Read the model definition and answer for the solid it produces. Units are mm, in the model's axes. A direction names the side the tool comes from. Coordinates: 2 decimals unless noted, no trailing zeros. Write each loop counter-clockwise with the first axis right and the second up, starting at its lowest first coordinate (ties: lowest second). Pieces come first, ordered by that corner, then holes.
(1) Find the intervals of material crossed by probe 1 along X at (y, z) = (34.5, -19.5); probe 2 along Z at (x, y) = (18.5, 43); probe 3 along X at (y, z) = (32, -22.5), in increasing order.
(2) Section C-C on y = 27 is taken. Write down the section's boundary in (x, z).
(3) Section A-A on y = -19 is taken. Write down the section's boundary in (x, z), then the cut area to 3 significant figures.
(4) Which of the six approach directions +Z, -Z, +X, -X, +Y, -Y give full straight-line access (tool end or side, diameter ignored) to faces 4 (the flat face through (11, -5, -36)), 5 (the flat face through (17.5, 0, 2)), 6 (the flat face through (22.56, 22.88, -23.2)), 7 (the cylindrical face through (12.99, -20.72, 1.52)), 8 (the flat face through (-1, 47, 13))?
(5) The mould has two halves that part along X. Classify faces 1 (the flat face through (50, 8, 1)), 2 (the flat face through (-17.5, 0, 2)), 3 (the flat face through (-50, 11, 2)): +X half, -X half, draft (parallel to the pull), parting line (faces both ways), or undercut.
(6) Section D-D on z = -21 is taken. Write down the section's boundary in (x, y).
(7) Section B-B on x = -15 is taken. Write down the section's boundary in (y, z), then the cut area to 3 significant figures.
(8) Given pin 1 (15 mm diameter, centred on x = 5, z = -36.5, fed in from -Y); pin 2 (10 mm diameter, centred on x = 22.5, z = 10.5, fed in from -Y); pin 3 (5 mm diameter, centred on x = -22.5, y = 15.5, fed in from -Z); pin 4 (12 mm diameter, centred on x = 18, z = -14.5, fed in from +Y), each flat-ended and moving along its own axis, determine where each tip first touches the part or whether it passes through.
Autodesk Inventor part; units mm, degrees
ref_plane "YZ Plane" through (0, 0, 0) normal (1, 0, 0) x (0, 1, 0)
ref_plane "XZ Plane" through (0, 0, 0) normal (0, 1, 0) x (-1, 0, 0)
ref_plane "XY Plane" through (0, 0, 0) normal (0, 0, 1) x (1, 0, 0)
sketch "Sketch1" plane through (0, 0, 0) normal (0, 0, 1) x (1, 0, 0)
  line L0 (-50, -50) -> (50, -50)
  line L1 (50, -50) -> (50, 50)
  line L2 (50, 50) -> (-50, 50)
  line L3 (-50, 50) -> (-50, -50)
  line L4 (-50, -50) -> (50, 50) construction
  line L5 (50, -50) -> (-50, 50) construction
  point P0 (0, 0)
  dimension "d0" = 100
  dimension "d1" = 100
extrude "Extrusion1" add sketch "Sketch1" along normal blind 3
sketch "Sketch2" plane through (-50, 50, 0) normal (0, 1, 0) x (1, 0, 0)
  line L0 (0, 0) -> (100, 0)
  line L1 (0, 0) -> (50, 50)
  line L2 (50, 50) -> (52.1213, 47.8787)
  line L3 (52.1213, 47.8787) -> (2.1213, -2.1213)
  line L4 (2.1213, -2.1213) -> (0, 0)
  line L5 (0, 0) -> (70.7107, 0) construction
  line L6 (100, 0) -> (52.1213, 47.8787)
  line L7 (52.1213, 47.8787) -> (50, 45.7574)
  line L8 (50, 45.7574) -> (97.8787, -2.1213)
  line L9 (97.8787, -2.1213) -> (100, 0)
  point P0 (50, 0)
  dimension "d4" = 45
  dimension "d5" = 3
  dimension "d6" = 3
extrude "Extrusion2" add sketch "Sketch2" against normal blind 55 contours L1 L2 L3 L0 | L0 L3 L4 | L8 L3 L6 L0 | L0 L9 L8
sketch "Sketch3" plane through (0, 0, 3) normal (0, 0, 1) x (1, 0, 0)
  line L0 (2.5, -25) -> (-2.5, -25)
  line L1 (-17.5, -10) -> (-17.5, 10)
  line L2 (-2.5, 25) -> (2.5, 25)
  line L3 (17.5, 10) -> (17.5, -10)
  line L4 (17.5, -25) -> (-17.5, 25) construction
  line L5 (-17.5, -25) -> (17.5, 25) construction
  arc A0 (-2.5, 25) -> (-17.5, 10) centre (-2.5, 10) ccw
  arc A1 (17.5, 10) -> (2.5, 25) centre (2.5, 10) ccw
  arc A2 (2.5, -25) -> (17.5, -10) centre (2.5, -10) ccw
  arc A3 (-17.5, -10) -> (-2.5, -25) centre (-2.5, -10) ccw
  point P0 (0, 0)
  dimension "d9" = 35
  dimension "d10" = 50
  dimension "d11" = 15
extrude "Extrusion3" cut sketch "Sketch3" against normal blind 3
sketch "Sketch5" plane through (-50, 50, 3) normal (0, 1, 0) x (1, 0, 0)
  line L0 (0, 3) -> (0, 0)
  line L1 (0, 0) -> (100, 0)
  line L2 (100, 0) -> (100, -20)
  line L3 (100, -20) -> (0, -20)
  line L4 (0, -20) -> (0, 0)
  point P0 (50, 3)
  dimension "d16" = 100
  dimension "d17" = 20
extrude "Extrusion5" add sketch "Sketch5" against normal blind 3
properties part number "fixation_v02"
Response:
1. probe 1: x = -30.5 to -26.26, 26.26 to 30.5
1. probe 2: z = -31.5 to -27.26, 0 to 3
1. probe 3: x = -27.5 to -23.26, 23.26 to 27.5
2. outline: (-50, 0) - (0, -50) - (50, 0) - (50, 3) - (-50, 3) - close; hole (-45.76, 0) - (0, -45.76) - (45.76, 0) - close
3. outline: (-50, 0) - (-14.5, 0) - (-14.5, 3) - (-50, 3) - close; (14.5, 0) - (50, 0) - (50, 3) - (14.5, 3) - close
3. area: 213 mm2
4. face 4: -Z, +X, -X, -Y
4. face 5: +Z
4. face 6: +Y, -Y
4. face 7: +Z, -Z
4. face 8: +Z, +X, -X, -Y
5. face 1: +X half
5. face 2: undercut
5. face 3: -X half
6. outline: (-29, -5) - (-24.76, -5) - (-24.76, 50) - (-29, 50) - close; (24.76, -5) - (29, -5) - (29, 50) - (24.76, 50) - close
7. outline: (-50, 0) - (-18.29, 0) - (-18.29, 3) - (-50, 3) - close; (-5, -35) - (50, -35) - (50, -30.76) - (-5, -30.76) - close; (18.29, 0) - (50, 0) - (50, 23) - (47, 23) - (47, 3) - (18.29, 3) - close
7. area: 484 mm2
8. pin 1: stops at y = -5
8. pin 2: stops at y = 47
8. pin 3: stops at z = -30
8. pin 4: passes through
